Geometry check sheet. Reference: drawing and pictorial views, mm from the part's lowest x, y, z. Coordinates: 2 decimals unless noted, no trailing zeros. Loops run counter-clockwise (first coordinate to the right, second up) from the corner with the lowest first, then second, coordinate; pieces in that order, holes last. Notation, with made-up numbers: M 49.5,-6 L 93.5,-6 A9 ccw 93.5,7 Z; hole C -25.75,56.25 d6. An arc over 180 degrees is marked long. Write each question's results on one line, items separated by ' | '. Start each with the question number.
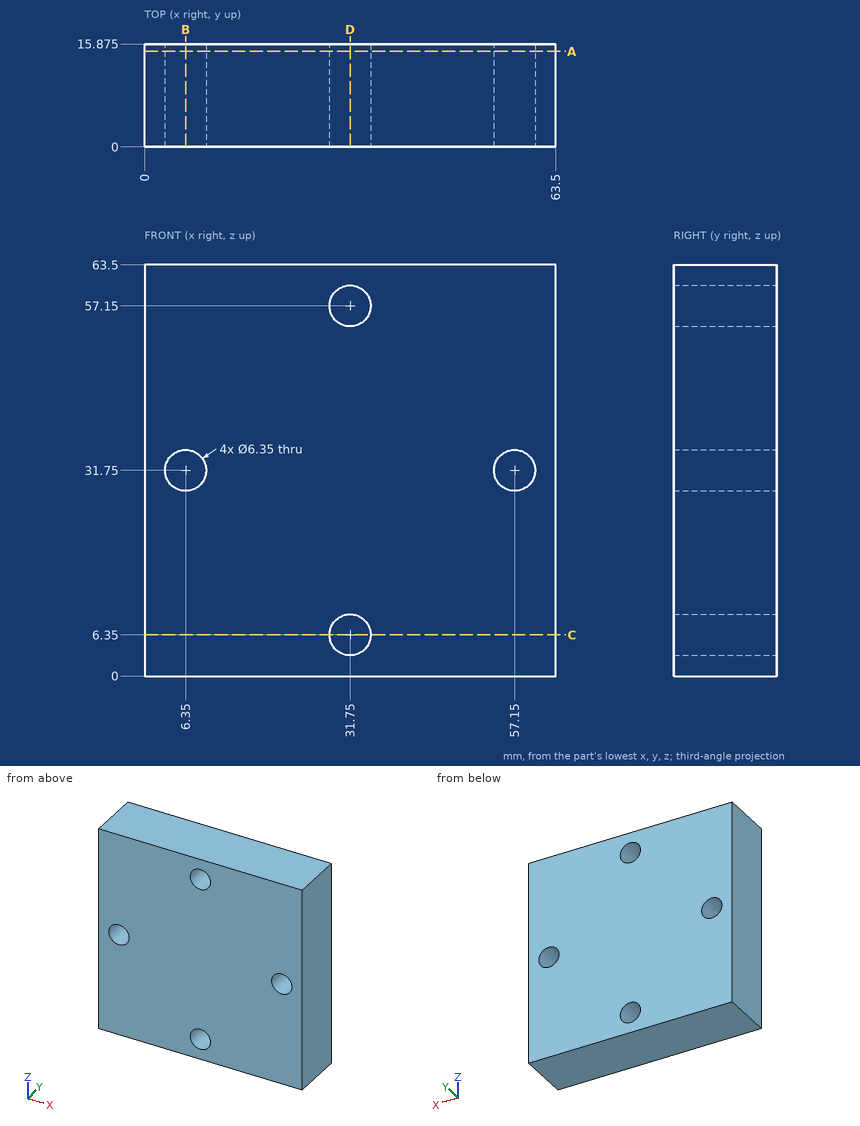
1) Gauge pin test, flat ends, axial feed: P1, Ø4, axis at x = 6.35, z = 31.75, coming from the +Y side; P2, Ø1.5, axis at x = 41.5, z = 9, coming from the -Y side. Record the tip position at first contact, or that the pin passes through.
2) Section check B-B (x = 6.35). Enter the section's corners in (y, z) (3 decimals).
3) Section check C-C (z = 6.35). Enter the section's corners in (x, y) (3 decimals), then the cut area to 3 significant figures.
4) Thickness scan on probe 1 along X at (y, z) = (8.5, 31.75) (3 decimals); probe 2 along Z at (x, y) = (6.35, 6.5) (3 decimals). Record the ranges inside material, lowest first.
5) Section check A-A (y = 14.75). Enter the section's corners in (x, z) (3 decimals).
6) Section check D-D (x = 31.75). Enter the section's corners in (y, z) (3 decimals), then the cut area to 3 significant figures.
Return value:
1) P1: passes through | P2: stops at y = 0
2) outline: M 0,0 L 15.875,0 L 15.875,28.575 L 0,28.575 Z; M 0,34.925 L 15.875,34.925 L 15.875,63.5 L 0,63.5 Z
3) outline: M 0,0 L 28.575,0 L 28.575,15.875 L 0,15.875 Z; M 34.925,0 L 63.5,0 L 63.5,15.875 L 34.925,15.875 Z | area: 907 mm2
4) probe 1: x = 0 to 3.175, 9.525 to 53.975, 60.325 to 63.5 | probe 2: z = 0 to 28.575, 34.925 to 63.5
5) outline: M 0,0 L 63.5,0 L 63.5,63.5 L 0,63.5 Z; hole C 6.35,31.75 d6.35; hole C 31.75,6.35 d6.35; hole C 31.75,57.15 d6.35; hole C 57.15,31.75 d6.35
6) outline: M 0,0 L 15.875,0 L 15.875,3.175 L 0,3.175 Z; M 0,9.525 L 15.875,9.525 L 15.875,53.975 L 0,53.975 Z; M 0,60.325 L 15.875,60.325 L 15.875,63.5 L 0,63.5 Z | area: 806 mm2
